Source: CAD feature listing. Evaluate the final solid. Frame: model axes, mm. Face numbers are marked on the shaded views. A direction names the side the tool comes from. Coordinates: 2 decimals unless noted, no trailing zeros. Order: outer loops, then holes, each group sorted by start corner. A loop starts at its lowest first (then second) coordinate and runs counter-clockwise, first axis right, second up.
Autodesk Inventor part; units mm, degrees
ref_plane "YZ Plane" through (0, 0, 0) normal (1, 0, 0) x (0, 1, 0)
ref_plane "XZ Plane" through (0, 0, 0) normal (0, 1, 0) x (-1, 0, 0)
ref_plane "XY Plane" through (0, 0, 0) normal (0, 0, 1) x (1, 0, 0)
sketch "Sketch1" plane through (0, 0, 0) normal (0, 0, 1) x (1, 0, 0)
  circle A0 centre (-15.5, 15.5) radius 1.75
  circle A1 centre (15.5, 15.5) radius 1.75
  circle A2 centre (-15.5, -15.5) radius 1.75
  circle A3 centre (15.5, -15.5) radius 1.75
  circle A4 centre (0, 0) radius 11.05
  line L0 (-15.5, 15.5) -> (15.5, 15.5) construction
  line L1 (15.5, 15.5) -> (15.5, -15.5) construction
  line L2 (15.5, -15.5) -> (-15.5, -15.5) construction
  line L3 (-15.5, -15.5) -> (-15.5, 15.5) construction
  line L4 (-15.5, 15.5) -> (15.5, -15.5) construction
  line L5 (15.5, 15.5) -> (-15.5, -15.5) construction
  line L6 (-25, 25) -> (-25, -25)
  line L7 (-25, -25) -> (25, -25)
  line L8 (25, -25) -> (25, 25)
  line L9 (25, 25) -> (-25, 25)
  dimension "d0" = 22.1
  dimension "d1" = 31
  dimension "d2" = 31
  dimension "d3" = 3.5
  dimension "d4" = 50
  dimension "d5" = 50
extrude "Extrusion1" add sketch "Sketch1" against normal blind 2
sketch "Sketch2" plane through (25, -25, 0) normal (1, 0, 0) x (0, 0, -1)
  line L0 (0, 0) -> (0, 50)
  line L1 (0, 0) -> (2, 0)
  line L2 (2, 50) -> (2, 0)
  line L3 (0, 50) -> (2, 50)
  line L4 (0, 0) -> (0, 50)
  line L5 (0, 60.1) -> (-17.583, 60.1)
  line L6 (-29.2887, 35.0756) -> (0, 0)
  line L7 (0, 38.75) -> (0, 42.25) construction
  line L8 (0, 44.85) -> (-34.6915, 44.85) construction
  line L9 (2, 50) -> (2, 60.1)
  line L10 (2, 60.1) -> (0, 60.1)
  circle A0 centre (-17.583, 44.85) radius 5
  circle A1 centre (-17.583, 44.85) radius 11.25
  circle A2 centre (-17.583, 44.85) radius 13.25
  arc A3 (-17.583, 60.1) -> (-29.2887, 35.0756) centre (-17.583, 44.85) ccw
  point P0 (0, 25)
  dimension "d8" = 19.85
  dimension "d9" = 19.583
  dimension "d10" = 10
  dimension "d11" = 22.5
  dimension "d12" = 2
  dimension "d13" = 2
extrude "Extrusion2" add sketch "Sketch2" against normal blind 7 contours L6 A3 L5 L10 L9 L3 L0 | A2
extrude "Extrusion3" add sketch "Sketch2" along normal blind 1 contours L6 A3 L5 L10 L9 L3 L0 | L0 L3 L2 L1 | A1 | A2
mirror "Mirror1" about plane through (0, 0, 0) normal (1, 0, 0) of "Extrusion2", "Extrusion3"
properties part number "Worm Gear Box" material "PC/ABS Plastic"
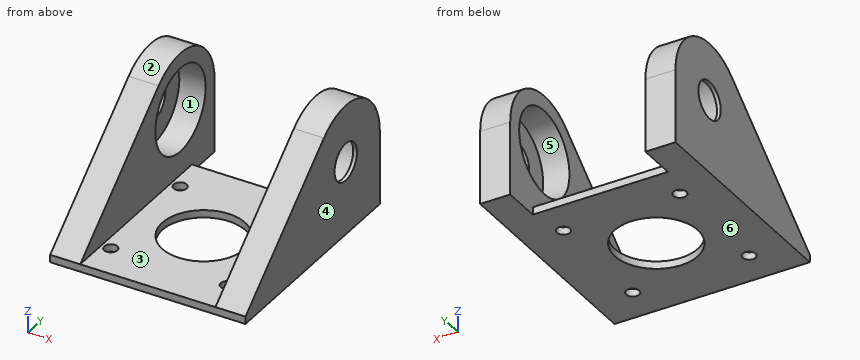
Q1. Section query A-A on x = 15.5. Output: boundary loops of the cut face in (y, z).
Solutions:
outline: (-25, -2) - (-17.25, -2) - (-17.25, 0) - (-25, 0) - close; (-13.75, -2) - (13.75, -2) - (13.75, 0) - (-13.75, 0) - close; (17.25, -2) - (25, -2) - (25, 0) - (17.25, 0) - close
Q2. Set-up query: the marked faces 1, 2 and 3. Return all of +Z, -Z, +X, -X, +Y, -Y with unobstructed straight access to the full face (end or side cutting, diameter ignored); none if empty.
Solutions:
face 1: none
face 2: +Z, +X, -X
face 3: +Z, +Y, -Y
Q3. Section query C-C on x = 8.5. Output: boundary loops of the cut face in (y, z).
Solutions:
outline: (-25, -2) - (-7.06, -2) - (-7.06, 0) - (-25, 0) - close; (7.06, -2) - (25, -2) - (25, 0) - (7.06, 0) - close
Q4. Pin query (flat end, axial travel): P1, Ø5.5, axis at x = -15.5, y = 15.5, coming from the -Z side; P2, Ø6, axis at x = -12.5, z = 11.5, coming from the -Y side; P3, Ø0.6, axis at x = -8, z = -1, coming from the +Y side; P4, Ø8, axis at x = -20, z = 27.5, coming from the +Y side. Return the tip coordinate at first contact, or that it passes through.
Solutions:
P1: stops at z = -2
P2: passes through
P3: stops at y = 25
P4: stops at y = 33.91
Q5. Section query D-D on z = 9.5. Output: boundary loops of the cut face in (x, y), plus the area to 3 significant figures.
Solutions:
outline: (-26, -13.62) - (-18, -13.62) - (-18, 12.03) - (-25, 12.03) - (-25, 27.67) - (-18, 27.67) - (-18, 35.1) - (-26, 35.1) - close; (18, -13.62) - (26, -13.62) - (26, 35.1) - (18, 35.1) - (18, 27.67) - (25, 27.67) - (25, 12.03) - (18, 12.03) - close
area: 560 mm2
Q6. Pull-direction query (X, two-part tool) for the marked faces 4, 5 and 6; classes: pulls with the +X half, pulls with the -X half, needs draft (parallel to the pull), parting line crosses it, or undercut.
Solutions:
face 4: pulls with the +X half
face 5: undercut
face 6: needs draft
Q7. Section query B-B on y = -8. Output: boundary loops of the cut face in (x, z), plus the area to 3 significant figures.
Solutions:
outline: (-26, -2) - (-7.62, -2) - (-7.62, 0) - (-18, 0) - (-18, 14.2) - (-26, 14.2) - close; (7.62, -2) - (26, -2) - (26, 14.2) - (18, 14.2) - (18, 0) - (7.62, 0) - close
area: 301 mm2
Q8. Material intervals for line 1 along Y through (x, z) = (15.5, -1.5); line 2 along X through (y, z) = (28, 6.5); line 3 along Y through (x, z) = (0, -0.35), sorted ascending.
Solutions:
line 1: y = -25 to -17.25, -13.75 to 13.75, 17.25 to 25
line 2: x = -26 to -18, 18 to 26
line 3: y = -25 to -11.05, 11.05 to 25
